from build123d import *

# Parameters (mm, degrees)
AUFSATZ_LINEAR_AUSTRAGEN1_DEPTH = 18
WANDUNG1_T                      = -2
SKIZZE2_R                       = 17.5
AUFSATZ_LINEAR_AUSTRAGEN2_DEPTH = 6


with BuildPart() as part:
    # Skizze1 → Aufsatz-Linear austragen1 (new body)
    with BuildSketch(Plane.XY):
        with BuildLine():
            Line((-30, -35), (30, -35))
            ThreePointArc((30, -35), (33.535533906, -33.535533906), (35, -30))
            Line((35, -30), (35, 30))
            ThreePointArc((35, 30), (33.535533906, 33.535533906), (30, 35))
            Line((30, 35), (-30, 35))
            ThreePointArc((-30, 35), (-33.535533906, 33.535533906), (-35, 30))
            Line((-35, 30), (-35, -30))
            ThreePointArc((-35, -30), (-33.535533906, -33.535533906), (-30, -35))
        make_face()
    extrude(amount=AUFSATZ_LINEAR_AUSTRAGEN1_DEPTH)

    # Wandung1
    wandung1_openings = [part.faces().sort_by_distance(p)[0] for p in [
        (0, 0, 0),
    ]]
    offset(amount=WANDUNG1_T, openings=wandung1_openings, kind=Kind.INTERSECTION)

    # Skizze2 → Aufsatz-Linear austragen2 (add)
    with BuildSketch(Plane.XY.offset(18)):
        Circle(SKIZZE2_R)
    extrude(amount=AUFSATZ_LINEAR_AUSTRAGEN2_DEPTH)

    # Skizze3 → Rotation1 (revolve)
    with BuildSketch(Plane(origin=(0, 0, 0), x_dir=(1, 0, 0), z_dir=(0, 1, 0))):
        with BuildLine():
            Line((0, -24), (37.5, -24))
            ThreePointArc((37.5, -24), (24.01171589, -45.577144863), (0, -54))
            Line((0, -54), (0, -24))
        make_face()
    revolve(axis=Axis((0, 0, -8.721924789), (0, 0, 1)))


solid = part.part
Can you work these out from the model? Positions are in its coordinate system, mm. A direction names the side the tool comes from. Give positions to 0.01 mm unless a question says otherwise; leave off trailing zeros. Loops run counter-clockwise (first coordinate to the right, second up) from the corner with the lowest first, then second, coordinate; pieces in that order, holes last. Notation, with made-up numbers: (-29.5, -6.75) - (16.5, -6.75) arc R26 cw to (16.5, 8.25) - close; hole circle Ø9 at (-4.5, 33). An arc over 180 degrees is marked (long way). Return JSON: item names as keys, results as strings.
1. I'm going to push flat-ended pins straight in: pin 1 Ø4 at (y, z) = (13.5, 6) entering from -X; pin 2 Ø5 at (y, z) = (11, 4.5) entering from +X; pin 3 Ø8 at (x, y) = (18.5, 15.5) entering from -Z. Where does each tip first touch, or does it pass through?
Output values:
{"pin 1": "stops at x = -35", "pin 2": "stops at x = 35", "pin 3": "stops at z = 16"}
2. I want a section at C-C on x = 0. Please give me the cut outline in (y, z) (1 decimal).
Output values:
{"outline": "(-37.5, 24) - (-17.5, 24) - (-17.5, 18) - (-35, 18) - (-35, 0) - (-33, 0) - (-33, 16) - (33, 16) - (33, 0) - (35, 0) - (35, 18) - (17.5, 18) - (17.5, 24) - (37.5, 24) arc R38.4 ccw to start"}
3. For faces 1 (the face through (0, -33, 8)), 2 (the face through (35, 0, 9)), 3 (the face through (-35, 0, 9)), which set-ups out of +Z, -Z, +X, -X, +Y, -Y let a thin tool reach every point of the face, with its end or its side?
Output values:
{"face 1": "-Z", "face 2": "-Z, +X, +Y, -Y", "face 3": "-Z, -X, +Y, -Y"}
4. I want a section at B-B on x = 26.5. Please give me the cut outline in (y, z), and give its area (3 significant figures).
Output values:
{"outline": "(-35, 0) - (-33, 0) - (-33, 16) - (33, 16) - (33, 0) - (35, 0) - (35, 18) - (-35, 18) - close; (-26.53, 24) - (26.53, 24) arc R27.84 ccw to start", "area": "959 mm²"}
5. If I drill on line 1 (X direction, y = -4, z = 5.5); line 2 (X direction, y = -24, z = 17.5); line 3 (Z direction, x = 27, y = -3.5), over which ranges is the centre line in solid material (lowest first)?
Output values:
{"line 1": "x = -35 to -33, 33 to 35", "line 2": "x = -35 to 35", "line 3": "z = 16 to 18, 24 to 42.7"}
6. We'd pull the mould along Z, two halves only. Please class faces 4 (the face through (0, 35, 9)), 5 (the face through (0, 0, 16)), 6 (the face through (-8, -16, 24)): +Z half, -Z half, draft (parallel to the pull), parting line (faces both ways), or undercut.
Output values:
{"face 4": "draft", "face 5": "-Z half", "face 6": "undercut"}
7. I want a section at A-A on z = 13. Please give me the cut outline in (x, y).
Output values:
{"outline": "(-35, -30) arc R5 ccw to (-30, -35) - (30, -35) arc R5 ccw to (35, -30) - (35, 30) arc R5 ccw to (30, 35) - (-30, 35) arc R5 ccw to (-35, 30) - close; hole (-33, -30) arc R3 ccw to (-30, -33) - (30, -33) arc R3 ccw to (33, -30) - (33, 30) arc R3 ccw to (30, 33) - (-30, 33) arc R3 ccw to (-33, 30) - close"}
